Could you check a few things on this drawing? It's one solid part, dimensions in mm from its lowest x, y, z. A direction names the side the tool comes from. Give positions to 0.01 mm unless a question says otherwise; leave off trailing zeros. Loops run counter-clockwise (first coordinate to the right, second up) from the corner with the lowest first, then second, coordinate; pieces in that order, holes last.
Q1. Suppose I cut it at A-A (y = 3.75). List the corners of the cut face in (x, z) for me, and give its area (3 significant figures).
Q2. Thinking about a two-plate mould opening in Z: for the marked faces 1, 2, 3 and 4, which applies, pulls with the +Z half, pulls with the -Z half, needs draft (parallel to the pull), parting line crosses it, or undercut?
Q3. Suppose I cut it at D-D (z = 27). List the corners of the cut face in (x, y) for me, and give its area (3 significant figures).
Q4. For the marked faces 5, 6 and 7, which set-ups out of +Z, -Z, +X, -X, +Y, -Y let a thin tool reach every point of the face, with its end or its side?
Q5. Suppose I cut it at C-C (x = 34). List the corners of the cut face in (y, z) for me, and give its area (3 significant figures).
Q6. I need wall thicknesses on probe 1 along Z at (x, y) = (30.5, 10); probe 2 along X at (y, z) = (11.5, 5); probe 3 along Z at (x, y) = (34, 5). Which ranges of each line are inside material? Lowest first, please.
Q7. I'm going to push flat-ended pins straight in: P1, Ø5, axis at y = 10, z = 23, coming from the -X side; P2, Ø2.5, axis at x = 35, z = 5, coming from the -Y side. Where does each tip first touch, or does it pass through?
Q8. Suppose I cut it at B-B (z = 5). List the corners of the cut face in (x, y) for me, and give its area (3 significant figures).
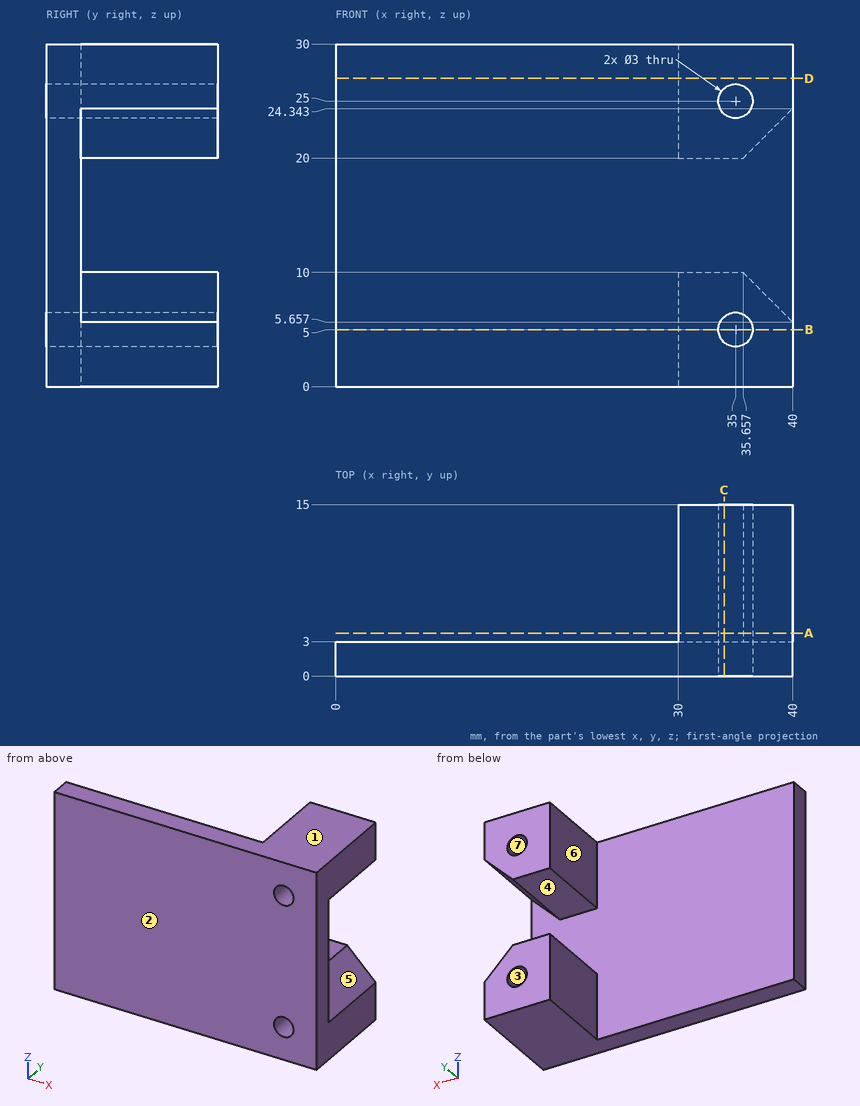
Solutions:
1. outline: (30, 0) - (40, 0) - (40, 5.66) - (35.66, 10) - (30, 10) - close; (30, 20) - (35.66, 20) - (40, 24.34) - (40, 30) - (30, 30) - close; hole circle Ø3 at (35, 5); hole circle Ø3 at (35, 25)
1. area: 167 mm2
2. face 1: pulls with the +Z half
2. face 2: needs draft
2. face 3: undercut
2. face 4: undercut
3. outline: (0, 0) - (40, 0) - (40, 15) - (30, 15) - (30, 3) - (0, 3) - close
3. area: 240 mm2
4. face 5: +X, +Y
4. face 6: +Z, -Z, -X, +Y
4. face 7: +Y, -Y
5. outline: (0, 0) - (15, 0) - (15, 3.88) - (0, 3.88) - close; (0, 6.12) - (15, 6.12) - (15, 10) - (3, 10) - (3, 20) - (15, 20) - (15, 23.88) - (0, 23.88) - close; (0, 26.12) - (15, 26.12) - (15, 30) - (0, 30) - close
5. area: 263 mm2
6. probe 1: z = 0 to 10, 20 to 30
6. probe 2: x = 30 to 33.5, 36.5 to 40
6. probe 3: z = 0 to 3.88, 6.12 to 10, 20 to 23.88, 26.12 to 30
7. P1: stops at x = 30
7. P2: passes through
8. outline: (0, 0) - (33.5, 0) - (33.5, 15) - (30, 15) - (30, 3) - (0, 3) - close; (36.5, 0) - (40, 0) - (40, 15) - (36.5, 15) - close
8. area: 195 mm2
